Geometry check sheet. Reference: the model listing, model coordinates, mm. Face numbers are marked on the shaded views. A direction names the side the tool comes from. Round coordinates to 2 decimals unless told otherwise and drop trailing zeros. Order: outer loops, then holes, each group sorted by start corner. A loop starts at its lowest first (then second) coordinate and runs counter-clockwise, first axis right, second up. Notation, with made-up numbers: (31, 6.25) - (37, 6.25) arc R14 ccw to (37, 28.25) - close; hole circle Ø4 at (45.25, 37). An arc over 180 degrees is marked (long way). Use a Markdown table: item, result. Add a question column.
(1) Thickness scan on line 1 along X through (y, z) = (3.75, -16); line 2 along Y through (x, z) = (48, -23.5); line 3 along X through (y, z) = (2, -27). Record the ranges inside material, lowest first. Write a range as [from, to].
(2) Section check A-A on z = -16. Record the boundary of the cut face in (x, y), then the cut area to 3 significant figures.
(3) Section check C-C on y = 20.5. Record the boundary of the cut face in (x, z).
(4) Access from +Z, -Z, +X, -X, +Y, -Y to the whole of each face (thin tool, end or side, straight path). Record for the marked faces 4, 5 and 6.
(5) Section check D-D on z = -23. Record the boundary of the cut face in (x, y), then the cut area to 3 significant figures.
(6) Section check B-B on x = 49.5. Record the boundary of the cut face in (y, z), then the cut area to 3 significant figures.
(7) Mould release check, pull along Y, two halves, no side actions. Record for the marked faces 1, 2 and 3: released by +Y, released by -Y, zero draft, split by the parting line, or undercut.
(8) Gauge pin test, flat ends, axial feed: P1, Ø5, axis at x = 30, z = -20.5, coming from the -Y side; P2, Ø1, axis at y = 25.5, z = -23, coming from the -X side; P3, Ø5.5, axis at x = 14.5, z = -19.5, coming from the +Y side; P4, Ø4, axis at x = 5, z = -16, coming from the +Y side. Record the tip position at first contact, or that the pin passes through.
```python
from build123d import *

# Parameters (mm, degrees)
SKETCH1_W           = 32
SKETCH1_H           = 32
BOSS_EXTRUDE1_DEPTH = 12
SKETCH3_R           = 9
CUT_EXTRUDE1_DEPTH  = 2
SKETCH5_R           = 3
CUT_EXTRUDE2_DEPTH  = 47.346520905
SKETCH6_R           = 1.7
CUT_EXTRUDE3_DEPTH  = 47.818799643
SKETCH7_W           = 32
SKETCH7_H           = 44
BOSS_EXTRUDE3_DEPTH = 20.152172572
SKETCH8_R           = 1.7
CUT_EXTRUDE4_DEPTH  = 64.118935352


with BuildPart() as part:
    # Sketch1 → Boss-Extrude1 (new body)
    with BuildSketch(Plane(origin=(0, 0, 0), x_dir=(1, 0, 0), z_dir=(0, 1, 0))):
        with Locations((16, 16)):
            Rectangle(SKETCH1_W, SKETCH1_H)
    extrude(amount=BOSS_EXTRUDE1_DEPTH)

    # Sketch3 → Cut-Extrude1 (cut)
    with BuildSketch(Plane(origin=(0, 12, 0), x_dir=(1, 0, 0), z_dir=(0, 1, 0))):
        with Locations(Location((16, 16, 0), (0, 0, 270))):
            Circle(SKETCH3_R)
    extrude(amount=-CUT_EXTRUDE1_DEPTH, mode=Mode.SUBTRACT)

    # Sketch5 → Cut-Extrude2 (cut, through all)
    with BuildSketch(Plane(origin=(0, 10, 0), x_dir=(1, 0, 0), z_dir=(0, 1, 0))):
        with Locations(Location((16, 16, 0), (0, 0, 270))):
            Circle(SKETCH5_R)
    extrude(amount=-CUT_EXTRUDE2_DEPTH, mode=Mode.SUBTRACT)

    # Sketch6 → Cut-Extrude3 (cut, through all)
    with BuildSketch(Plane(origin=(0, 12, 0), x_dir=(1, 0, 0), z_dir=(0, 1, 0))):
        with Locations(Location((16, 27, 0), (0, 0, 270))):
            Circle(SKETCH6_R)
        with Locations(Location((5, 16, 0), (0, 0, 270))):
            Circle(SKETCH6_R)
        with Locations(Location((16, 5, 0), (0, 0, 270))):
            Circle(SKETCH6_R)
        with Locations(Location((27, 16, 0), (0, 0, 270))):
            Circle(SKETCH6_R)
    extrude(amount=-CUT_EXTRUDE3_DEPTH, mode=Mode.SUBTRACT)

    # Sketch7 → Boss-Extrude3 (add)
    with BuildSketch(Plane(origin=(32, 0, 0), x_dir=(0, 0, -1), z_dir=(1, 0, 0))):
        with Locations((16, 22)):
            Rectangle(SKETCH7_W, SKETCH7_H)
    extrude(amount=BOSS_EXTRUDE3_DEPTH)

    # Sketch8 → Cut-Extrude4 (cut, through all)
    with BuildSketch(Plane.ZY.offset(-32)):
        with Locations((-23.5, 35.5)):
            Circle(SKETCH8_R)
        with Locations((-8.5, 35.5)):
            Circle(SKETCH8_R)
        with Locations((-8.5, 20.5)):
            Circle(SKETCH8_R)
        with Locations((-23.5, 20.5)):
            Circle(SKETCH8_R)
    extrude(amount=-CUT_EXTRUDE4_DEPTH, mode=Mode.SUBTRACT)


solid = part.part
```
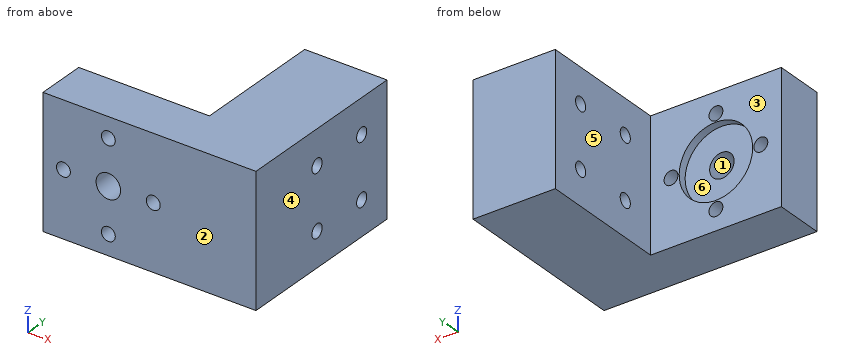
Check sheet entries:
| question | item | result |
|---|---|---|
| 1 | line 1 | x = [0, 3.3], [6.7, 13], [19, 25.3], [28.7, 52.15] |
| 1 | line 2 | y = [0, 18.8], [22.2, 33.8], [37.2, 44] |
| 1 | line 3 | x = [0, 14.3], [17.7, 52.15] |
| 2 | outline | (0, 0) - (3.3, 0) - (3.3, 12) - (0, 12) - close; (6.7, 0) - (13, 0) - (13, 10) - (7, 10) - (7, 12) - (6.7, 12) - close; (19, 0) - (25.3, 0) - (25.3, 12) - (25, 12) - (25, 10) - (19, 10) - close; (28.7, 0) - (52.15, 0) - (52.15, 44) - (32, 44) - (32, 12) - (28.7, 12) - close |
| 2 | area | 1,090 mm2 |
| 3 | outline | (32, -32) - (52.15, -32) - (52.15, -25.2) - (32, -25.2) - close; (32, -21.8) - (52.15, -21.8) - (52.15, -10.2) - (32, -10.2) - close; (32, -6.8) - (52.15, -6.8) - (52.15, 0) - (32, 0) - close |
| 4 | face 4 | +Z, -Z, +X, +Y, -Y |
| 4 | face 5 | +Z, -Z, -X, +Y |
| 4 | face 6 | +Y |
| 5 | outline | (0, 0) - (52.15, 0) - (52.15, 18.88) - (32, 18.88) - (32, 12) - (21.66, 12) - (21.66, 10) - (10.34, 10) - (10.34, 12) - (0, 12) - close; (32, 22.12) - (52.15, 22.12) - (52.15, 33.88) - (32, 33.88) - close; (32, 37.12) - (52.15, 37.12) - (52.15, 44) - (32, 44) - close |
| 5 | area | 1,120 mm2 |
| 6 | outline | (0, -32) - (44, -32) - (44, 0) - (0, 0) - close; hole circle Ø3.4 at (20.5, -23.5); hole circle Ø3.4 at (20.5, -8.5); hole circle Ø3.4 at (35.5, -23.5); hole circle Ø3.4 at (35.5, -8.5) |
| 6 | area | 1,370 mm2 |
| 7 | face 1 | zero draft |
| 7 | face 2 | released by -Y |
| 7 | face 3 | released by +Y |
| 8 | P1 | stops at y = 0 |
| 8 | P2 | stops at x = 32 |
| 8 | P3 | stops at y = 10 |
| 8 | P4 | stops at y = 12 |
